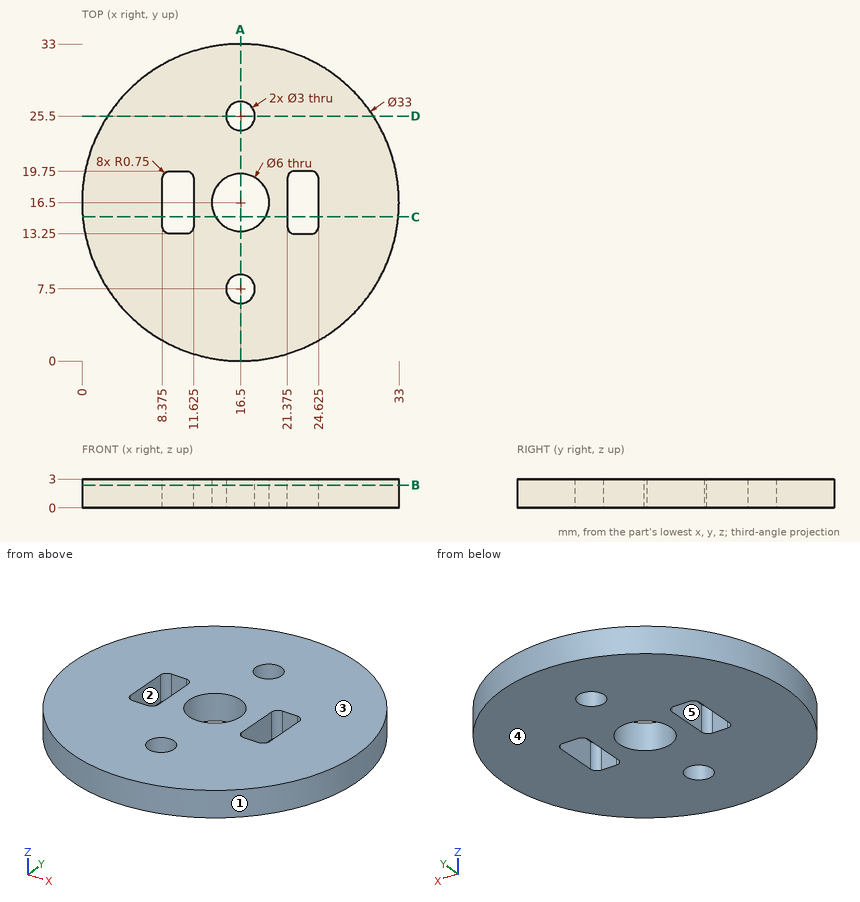
Study the drawing (mm; zero at the part's minimum x, y, z) and answer. A direction names the side the tool comes from. Round coordinates to 2 decimals unless told otherwise and drop trailing zeros. Write each loop counter-clockwise with the first axis right and the second up, starting at its lowest first coordinate (ties: lowest second). Pieces come first, ordered by that corner, then holes. Notation, with made-up numbers: (2, 68) -> (6, 68) arc R7 cw to (6, 78) -> close; hole circle Ø2 at (27.25, 21). An arc over 180 degrees is marked (long way). Use CSV: the item, a comma, the result in double quotes. Start each with the question number.
(1) Section B-B on z = 2.35 is taken. Give the vertices of the cut face in (x, y) (3 decimals), then the cut area to 3 significant figures.
(2) Which of the six approach directions +Z, -Z, +X, -X, +Y, -Y give full straight-line access (tool end or side, diameter ignored) to the marked faces 4 and 5?
(3) Section A-A on x = 16.5 is taken. Give the vertices of the cut face in (y, z), then the cut area to 3 significant figures.
(4) Each of these flat-tipped pins is pushed along its axis until it touches: pin 1 (1.5 mm diameter, centred on y = 15.5, z = 2, fed in from +X); pin 2 (0.5 mm diameter, centred on x = 10, z = 1.5, fed in from +Y); pin 3 (0.5 mm diameter, centred on x = 23.5, z = 2, fed in from -Y). Where does it stop, or does it pass through?
(5) Section C-C on y = 15 is taken. Give the vertices of the cut face in (x, z) (3 decimals).
(6) Consider L1, parallel to Y at x = 16.5, z = 1; L2, parallel to X at y = 26.5, z = 1.2; L3, parallel to X at y = 25.5, z = 2.6. Determine where each line is inside the solid, lowest interval first. Write a range as from..to.
(7) The mould has two halves that part along X. Classify the marked faces 1, 2 and 3: released by +X, released by -X, zero draft, split by the parting line, or undercut.
(8) Section D-D on y = 25.5 is taken. Give the vertices of the cut face in (x, z).
A:
1,outline,"circle Ø33 at (16.5, 16.5); hole (8.375, 14) arc R0.75 ccw to (9.125, 13.25) -> (10.875, 13.25) arc R0.75 ccw to (11.625, 14) -> (11.625, 19) arc R0.75 ccw to (10.875, 19.75) -> (9.125, 19.75) arc R0.75 ccw to (8.375, 19) -> close; hole circle Ø6 at (16.5, 16.5); hole circle Ø3 at (16.5, 7.5); hole circle Ø3 at (16.5, 25.5); hole (21.375, 14) arc R0.75 ccw to (22.125, 13.25) -> (23.875, 13.25) arc R0.75 ccw to (24.625, 14) -> (24.625, 19) arc R0.75 ccw to (23.875, 19.75) -> (22.125, 19.75) arc R0.75 ccw to (21.375, 19) -> close"
1,area,"772 mm²"
2,face 4,"-Z, +X, -X, +Y, -Y"
2,face 5,"+Z, -Z"
3,outline,"(0, 0) -> (6, 0) -> (6, 3) -> (0, 3) -> close; (9, 0) -> (13.5, 0) -> (13.5, 3) -> (9, 3) -> close; (19.5, 0) -> (24, 0) -> (24, 3) -> (19.5, 3) -> close; (27, 0) -> (33, 0) -> (33, 3) -> (27, 3) -> close"
3,area,"63.0 mm²"
4,pin 1,"stops at x = 33"
4,pin 2,"stops at y = 31.77"
4,pin 3,"stops at y = 1.44"
5,outline,"(0.068, 0) -> (8.375, 0) -> (8.375, 3) -> (0.068, 3) -> close; (11.625, 0) -> (13.902, 0) -> (13.902, 3) -> (11.625, 3) -> close; (19.098, 0) -> (21.375, 0) -> (21.375, 3) -> (19.098, 3) -> close; (24.625, 0) -> (32.932, 0) -> (32.932, 3) -> (24.625, 3) -> close"
6,L1,"y = 0..6, 9..13.5, 19.5..24, 27..33"
6,L2,"x = 3.38..15.38, 17.62..29.62"
6,L3,"x = 2.67..15, 18..30.33"
7,face 1,"split by the parting line"
7,face 2,"undercut"
7,face 3,"zero draft"
8,outline,"(2.67, 0) -> (15, 0) -> (15, 3) -> (2.67, 3) -> close; (18, 0) -> (30.33, 0) -> (30.33, 3) -> (18, 3) -> close"
